The figure shows three views and two pictorial views of one solid part (mm, origin at its lowest corner). Answer the questions. A direction names the side the tool comes from. Round coordinates to 2 decimals unless told otherwise and drop trailing zeros. Write each loop counter-clockwise with the first axis right and the second up, starting at its lowest first coordinate (ties: lowest second). Pieces come first, ordered by that corner, then holes.
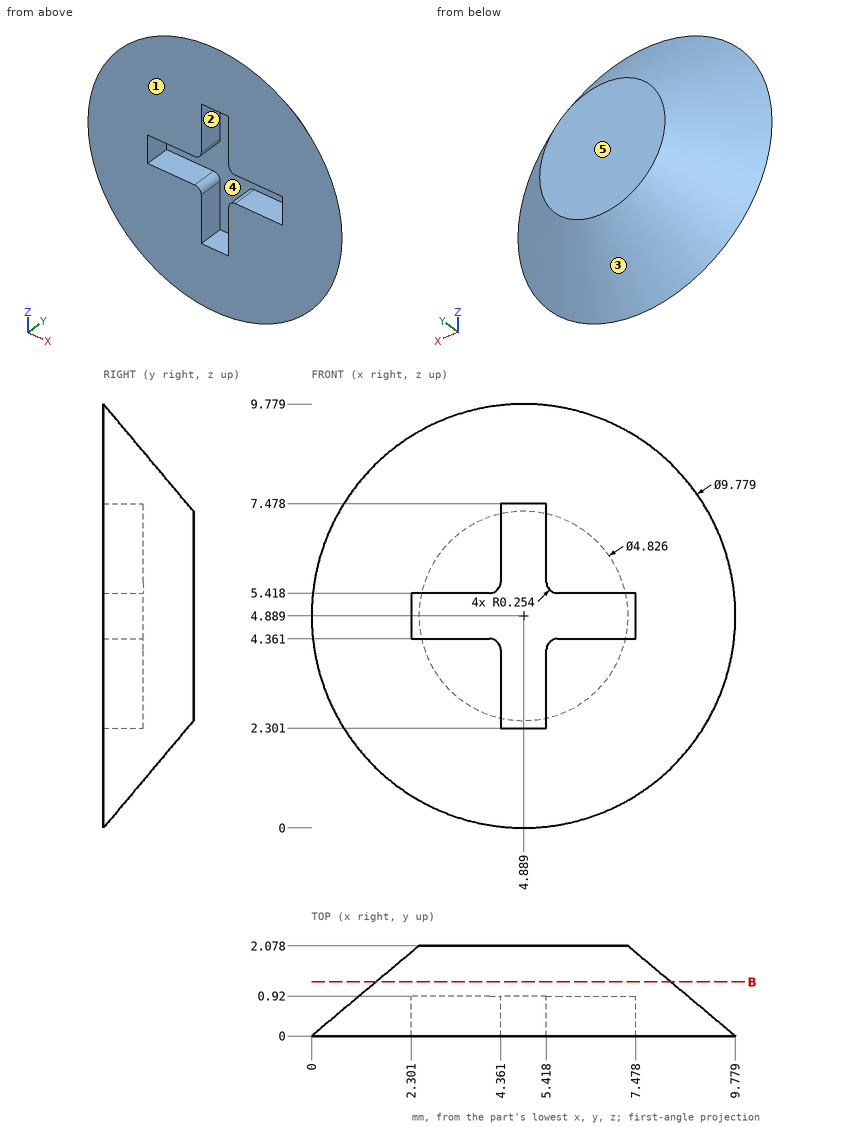
Q1. Flat-ended cylindrical pins translate along their axes: pin 1 Ø0.5 at (y, z) = (0.5, 3) entering from -X (1 decimal); pin 2 Ø1 at (x, y) = (3, 0.5) entering from -Z; pin 3 Ø1 at (x, y) = (3.5, 0.5) entering from +Z (1 decimal). Find the tip coordinate at first contact, or state that the pin passes through.
Verdict:
pin 1: stops at x = 0.7
pin 2: stops at z = 0.35
pin 3: stops at z = 9.6
Q2. Straight lines are drawn through the part: probe 1 along X at (y, z) = (0.8, 3) (1 decimal); probe 2 along Z at (x, y) = (6.75, 0.65) (1 decimal); probe 3 along X at (y, z) = (0.1, 3) (1 decimal). For each, find the intervals that lie inside material, in ascending order.
Verdict:
probe 1: x = 1.4 to 4.4, 5.4 to 8.3
probe 2: z = 1.2 to 4.4, 5.4 to 8.6
probe 3: x = 0.5 to 4.4, 5.4 to 9.3
Q3. Section B-B (y = 1.25) is taken. Determine the outline of the cut face in (x, z).
Verdict:
outline: circle Ø6.8 at (4.89, 4.89)
Q4. Which of the six approach directions +Z, -Z, +X, -X, +Y, -Y give full straight-line access (tool end or side, diameter ignored) to the marked faces 4 and 5?
Verdict:
face 4: -Y
face 5: +Z, -Z, +X, -X, +Y
Q5. Determine the mould class of the marked faces 1, 2 and 3 for opening direction X: pulls with the +X half, pulls with the -X half, needs draft (parallel to the pull), parting line crosses it, or undercut.
Verdict:
face 1: needs draft
face 2: undercut
face 3: parting line crosses it
